from build123d import *

# Parameters (mm, degrees)
SKETCH1_R           = 11
BOSS_EXTRUDE1_DEPTH = 25
SKETCH2_R           = 4
CUT_EXTRUDE1_DEPTH  = 30.444863729
CUT_EXTRUDE2_DEPTH  = 7.5
SKETCH4_R           = 1.5
CUT_EXTRUDE3_DEPTH  = 30.444863729
SKETCH5_R           = 1.5
CUT_EXTRUDE4_DEPTH  = 30.444863896
CUT_EXTRUDE5_START  = -10.2
SKETCH7_R           = 2.1
CUT_EXTRUDE5_DEPTH  = 10
CUT_EXTRUDE6_START  = -10.2
SKETCH8_R           = 2.1
CUT_EXTRUDE6_DEPTH  = 10


with BuildPart() as part:
    # Sketch1 → Boss-Extrude1 (new body)
    with BuildSketch(Plane(origin=(0, 0, 0), x_dir=(1, 0, 0), z_dir=(0, 1, 0))):
        with Locations(Location((0, 0, 0), (0, 0, 270))):
            Circle(SKETCH1_R)
    extrude(amount=BOSS_EXTRUDE1_DEPTH)

    # Sketch2 → Cut-Extrude1 (cut, through all)
    with BuildSketch(Plane(origin=(0, 25, 0), x_dir=(1, 0, 0), z_dir=(0, 1, 0))):
        with Locations(Location((0, 0, 0), (0, 0, 270))):
            Circle(SKETCH2_R)
    extrude(amount=-CUT_EXTRUDE1_DEPTH, mode=Mode.SUBTRACT)

    # Sketch3 → Cut-Extrude2 (cut)
    with BuildSketch(Plane.XZ):
        with BuildLine():
            Line((4.864454926, 3.520952041), (6.505382387, 5.161879503))
            Line((6.505382387, 5.161879503), (5.161879503, 6.505382387))
            Line((5.161879503, 6.505382387), (3.520952041, 4.864454926))
            ThreePointArc((3.520952041, 4.864454926), (2.298014011, 5.547896593), (0.95, 5.929378129))
            Line((0.95, 5.929378129), (0.95, 8.25))
            Line((0.95, 8.25), (-0.95, 8.25))
            Line((-0.95, 8.25), (-0.95, 5.929378129))
            ThreePointArc((-0.95, 5.929378129), (-2.298014011, 5.547896593), (-3.520952041, 4.864454926))
            Line((-3.520952041, 4.864454926), (-5.161879503, 6.505382387))
            Line((-5.161879503, 6.505382387), (-6.505382387, 5.161879503))
            Line((-6.505382387, 5.161879503), (-4.864454926, 3.520952041))
            ThreePointArc((-4.864454926, 3.520952041), (-5.547896593, 2.298014011), (-5.929378129, 0.95))
            Line((-5.929378129, 0.95), (-8.25, 0.95))
            Line((-8.25, 0.95), (-8.25, -0.95))
            Line((-8.25, -0.95), (-5.929378129, -0.95))
            ThreePointArc((-5.929378129, -0.95), (-5.547896593, -2.298014011), (-4.864454926, -3.520952041))
            Line((-4.864454926, -3.520952041), (-6.505382387, -5.161879503))
            Line((-6.505382387, -5.161879503), (-5.161879503, -6.505382387))
            Line((-5.161879503, -6.505382387), (-3.520952041, -4.864454926))
            ThreePointArc((-3.520952041, -4.864454926), (-2.298014011, -5.547896593), (-0.95, -5.929378129))
            Line((-0.95, -5.929378129), (-0.95, -8.25))
            Line((-0.95, -8.25), (0.95, -8.25))
            Line((0.95, -8.25), (0.95, -5.929378129))
            ThreePointArc((0.95, -5.929378129), (2.298014011, -5.547896593), (3.520952041, -4.864454926))
            Line((3.520952041, -4.864454926), (5.161879503, -6.505382387))
            Line((5.161879503, -6.505382387), (6.505382387, -5.161879503))
            Line((6.505382387, -5.161879503), (4.864454926, -3.520952041))
            ThreePointArc((4.864454926, -3.520952041), (5.547896593, -2.298014011), (5.929378129, -0.95))
            Line((5.929378129, -0.95), (8.25, -0.95))
            Line((8.25, -0.95), (8.25, 0.95))
            Line((8.25, 0.95), (5.929378129, 0.95))
            ThreePointArc((5.929378129, 0.95), (5.547896593, 2.298014011), (4.864454926, 3.520952041))
        make_face()
    extrude(amount=-CUT_EXTRUDE2_DEPTH, mode=Mode.SUBTRACT)

    # Sketch4 → Cut-Extrude3 (cut, through all)
    with BuildSketch(Plane.XY):
        with Locations((0, 19)):
            Circle(SKETCH4_R)
    extrude(amount=-CUT_EXTRUDE3_DEPTH, mode=Mode.SUBTRACT)

    # Sketch5 → Cut-Extrude4 (cut, through all)
    with BuildSketch(Plane(origin=(0, 0, 0), x_dir=(0, 0, -1), z_dir=(1, 0, 0))):
        with Locations((0, 19)):
            Circle(SKETCH5_R)
    extrude(amount=-CUT_EXTRUDE4_DEPTH, mode=Mode.SUBTRACT)

    # Sketch7 → Cut-Extrude5 (cut)
    with BuildSketch(Plane.XY.offset(CUT_EXTRUDE5_START)):
        with Locations((0, 19)):
            Circle(SKETCH7_R)
    extrude(amount=-CUT_EXTRUDE5_DEPTH, mode=Mode.SUBTRACT)

    # Sketch8 → Cut-Extrude6 (cut)
    with BuildSketch(Plane(origin=(0, 0, 0), x_dir=(0, 0, -1), z_dir=(1, 0, 0)).offset(CUT_EXTRUDE6_START)):
        with Locations((0, 19)):
            Circle(SKETCH8_R)
    extrude(amount=-CUT_EXTRUDE6_DEPTH, mode=Mode.SUBTRACT)


solid = part.part
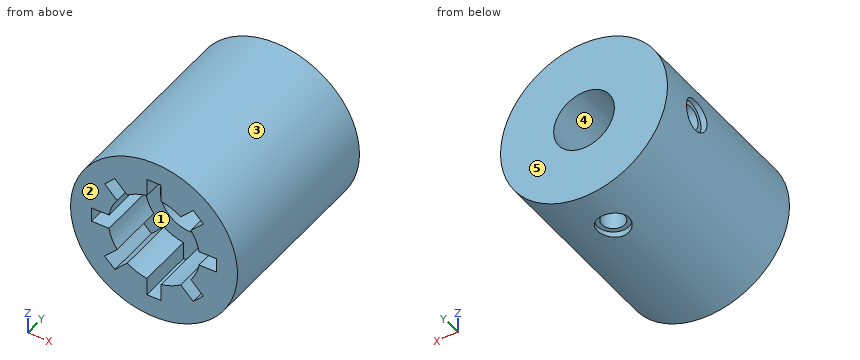
The model under review builds one solid part; all positions refer to its coordinate system, in mm. Face numbers are marked on the shaded views. A direction names the side the tool comes from. Give positions to 0.01 mm unless a question says otherwise; leave off trailing zeros. Order: outer loops, then holes, each group sorted by start corner. A loop starts at its lowest first (then second) coordinate and runs counter-clockwise, first axis right, second up. Notation, with made-up numbers: (-11.75, 38.25) -> (47.25, 38.25) arc R33 ccw to (47.25, 66.25) -> close; hole circle Ø8 at (60.25, -14.75). An arc over 180 degrees is marked (long way). Write item = value, one per line. Start each with the question number.
(1) Take a section at D-D (z = -3). Write out the cut boundary in (x, y), plus the area to 3 significant figures.
(2) Tool access review of the marked faces 1 and 2: name each direction out of +Z, -Z, +X, -X, +Y, -Y from which nothing blocks a thin tool from reaching the whole face with its end or side.
(3) Take a section at A-A (x = 0). Write out the cut boundary in (y, z), plus the area to 3 significant figures.
(4) For L1, parallel to Z at x = 0, y = 20.75; L2, parallel to Y at x = -7.5, z = 0; L3, parallel to Z at x = 0, y = 11.5, list the stretches that pass through material, from the lowest coordinate up. Write a range as from..to.
(5) For pin 1 Ø4 at (x, y) = (-5.5, 19) entering from +Z; pin 2 Ø4 at (y, z) = (13.5, -8.5) entering from -X; pin 3 Ø1.8 at (y, z) = (19, 0) entering from -X; pin 4 Ø7 at (x, z) = (0, 0) entering from -Y, all flat-tipped, find the tip position at first contact; note any pin that passes through.
(6) Draft analysis for pull direction X (two halves, no side actions). For the marked faces 3, 4 and 5, state which applies: +X half, -X half, draft (parallel to the pull), parting line (faces both ways), or undercut.
(7) Take a section at C-C (z = 0). Write out the cut boundary in (x, y), plus the area to 3 significant figures.
Returned:
q1.outline = (-10.58, 0) -> (-5.2, 0) -> (-5.2, 7.5) -> (-2.65, 7.5) -> (-2.65, 25) -> (-10.58, 25) -> close; (2.65, 7.5) -> (5.2, 7.5) -> (5.2, 0) -> (10.58, 0) -> (10.58, 25) -> (2.65, 25) -> close
q1.area = 359 mm²
q2.face_1 = -Y
q2.face_2 = +Z, -Z, +X, -X, -Y
q3.outline = (0, -11) -> (16.9, -11) -> (16.9, -10.2) -> (17.5, -10.2) -> (17.5, -4) -> (7.5, -4) -> (7.5, -8.25) -> (0, -8.25) -> close; (0, 8.25) -> (7.5, 8.25) -> (7.5, 4) -> (25, 4) -> (25, 11) -> (0, 11) -> close; (20.5, -10.2) -> (21.1, -10.2) -> (21.1, -11) -> (25, -11) -> (25, -4) -> (20.5, -4) -> close
q3.area = 264 mm²
q4.L1 = -10.2..-4, 4..11
q4.L2 = 7.5..17.5, 20.5..25
q4.L3 = -11..-4, 4..11
q5.pin_1 = 10.43
q5.pin_2 = -8.87
q5.pin_3 = 3.9
q5.pin_4 = through
q6.face_3 = parting line
q6.face_4 = undercut
q6.face_5 = draft
q7.outline = (-11, 0) -> (-8.25, 0) -> (-8.25, 7.5) -> (-4, 7.5) -> (-4, 17.5) -> (-10.2, 17.5) -> (-10.2, 16.9) -> (-11, 16.9) -> close; (-11, 21.1) -> (-10.2, 21.1) -> (-10.2, 20.5) -> (-4, 20.5) -> (-4, 25) -> (-11, 25) -> close; (4, 7.5) -> (8.25, 7.5) -> (8.25, 0) -> (11, 0) -> (11, 25) -> (4, 25) -> close
q7.area = 264 mm²
